Read the model definition and answer for the solid it produces. Units are mm, in the model's axes. A direction names the side the tool comes from. Coordinates: 2 decimals unless noted, no trailing zeros. Order: outer loops, then holes, each group sorted by start corner. A loop starts at its lowest first (then second) coordinate and runs counter-clockwise, first axis right, second up.
```python
from build123d import *

# Parameters (mm, degrees)
F1_DEPTH  = 38.1
F2_DEPTH  = 469.9
F3_DEPTH  = 469.9
F4_DEPTH  = 469.9
F6_DEPTH  = 25.4
F8_DEPTH  = 127
F9_R      = 254
F10_DEPTH = 38.1
F12_DEPTH = 38.1


with BuildPart() as f1:
    # F0 (on Top) → F1 (new body)
    with BuildSketch(Plane.XY):
        Polygon((-164.0508631923, -164.0508649307), (-200.8490917777, -173.9250926458), (-173.9250929642, -200.8490929642), align=None)
        Polygon((-173.9250929642, -200.8490929642), (-200.8490917777, -173.9250926458), (-317.5924246142, -290.6684189572), (-290.6851930936, -317.6091865675), align=None)
        Polygon((-243.6374118769, -14.4661021088), (-200.8490917777, -173.9250926458), (-164.0508631923, -164.0508649307), (-206.8391832914, -4.5918743936), align=None)
        Polygon((-164.0508631923, -164.0508649307), (-173.9250929642, -200.8490929642), (-14.4661048188, -243.6374219761), (-4.5918750468, -206.8391939425), align=None)
        Polygon((-290.6851930936, -317.6091865675), (-317.5924246142, -290.6684189572), (-344.5331937303, -317.6091865675), (-317.6259622097, -344.5499541778), align=None)
        Polygon((-253.5116395921, 22.3321264767), (-243.6374118769, -14.4661021088), (-206.8391832914, -4.5918743936), (-216.7134110066, 32.2063541919), align=None)
        Polygon((-4.5918750468, -206.8391939425), (-14.4661048188, -243.6374219761), (22.3321232148, -253.5116517481), (32.2063529868, -216.7134237145), align=None)
    extrude(amount=-F1_DEPTH)

    # F0 (on Top) → F2 (join)
    with BuildSketch(Plane.XY):
        Polygon((-290.6851930936, -317.6091865675), (-317.5924246142, -290.6684189572), (-344.5331937303, -317.6091865675), (-317.6259622097, -344.5499541778), align=None)
    extrude(amount=F2_DEPTH)

    # F0 (on Top) → F3 (join)
    with BuildSketch(Plane.XY):
        Polygon((-4.5918750468, -206.8391939425), (-14.4661048188, -243.6374219761), (22.3321232148, -253.5116517481), (32.2063529868, -216.7134237145), align=None)
    extrude(amount=F3_DEPTH)

    # F0 (on Top) → F4 (join)
    with BuildSketch(Plane.XY):
        Polygon((-253.5116395921, 22.3321264767), (-243.6374118769, -14.4661021088), (-206.8391832914, -4.5918743936), (-216.7134110066, 32.2063541919), align=None)
    extrude(amount=F4_DEPTH)

    # F5 (on face) → F6 (join)
    with BuildSketch(Plane.XY.offset(469.9)):
        with BuildLine():
            Line((75.3796231443, -162.8212069793), (-156.5023640677, 72.2591707782))
            ThreePointArc((-156.5023640677, 72.2591707782), (-358.8121384382, -359.2018192073), (75.3796231443, -162.8212069793))
        make_face()
    extrude(amount=F6_DEPTH)

    # F7 (on face) → F8 (join)
    with BuildSketch(Plane.XY.offset(495.3)):
        with BuildLine():
            Line((75.3796231443, -162.8212069793), (-199.4597931818, -433.9212904052))
            ThreePointArc((-199.4597931818, -433.9212904052), (0.3896807691, -361.662119627), (75.3796231443, -162.8212069793))
        make_face()
        with BuildLine():
            ThreePointArc((-156.5023640677, 72.2591707782), (-356.3518380185, 0), (-431.3417803937, -198.8409126477))
            Line((-431.3417803937, -198.8409126477), (-156.5023640677, 72.2591707782))
        make_face()
    extrude(amount=F8_DEPTH)

    # F9 (on face) → F10 (join)
    with BuildSketch(Plane.XY.offset(622.3)):
        with Locations((-177.9810786247, -180.8310598135)):
            Circle(F9_R)
    extrude(amount=F10_DEPTH)

    # F11 (on face) → F12 (cut)
    with BuildSketch(Plane.XY.offset(660.4)):
        with BuildLine():
            ThreePointArc((75.3308407052, -162.1476038864), (2.7361824332, -2.3450055803), (-156.1522700542, 72.2292158451))
            Line((-156.1522700542, 72.2292158451), (75.3308407052, -162.1476038864))
        make_face()
    extrude(amount=-F12_DEPTH, mode=Mode.SUBTRACT)


solid = f1.part
```
1) Which of the six approach directions +Z, -Z, +X, -X, +Y, -Y give full straight-line access (tool end or side, diameter ignored) to faces 5 (the flat face through (-244.857, -9.919, 158.27)), 6 (the flat face through (-10.84, -244.61, 158.27)), 7 (the flat face through (-9.46, -224.98, 231.66))?
A:
face 5: -Z, -X
face 6: -Z, -Y
face 7: -X, +Y
2) A cutting plane is placed at A-A, the plane z = 393. Determine the outline of the cut face in (x, y).
A:
outline: (-344.53, -317.61) - (-317.63, -344.55) - (-290.69, -317.61) - (-317.59, -290.67) - close; (-253.51, 22.33) - (-243.64, -14.47) - (-206.84, -4.59) - (-216.71, 32.21) - close; (-14.47, -243.64) - (22.33, -253.51) - (32.21, -216.71) - (-4.59, -206.84) - close
3) Straight lines are drawn through the part: line 1 (Z direction, x = -318.5, y = -339.5); line 2 (Z direction, x = -23, y = -180); line 3 (Z direction, x = 0, y = -273.5). For each, find the intervals that lie inside material, in ascending order.
A:
line 1: z = -38.1 to 495.3, 622.3 to 660.4
line 2: z = 469.9 to 495.3, 622.3 to 660.4
line 3: z = 469.9 to 660.4
4) Determine the mould class of faces 1 (the flat face through (-182, -177, 660.4)), 2 (the flat face through (-295.85, -65.19, 557.91)), 3 (the flat face through (-182, -177, 495.3)), 4 (the flat face through (-38.938, -46.927, 482.422)) for opening direction Z: pulls with the +Z half, pulls with the -Z half, needs draft (parallel to the pull), parting line crosses it, or undercut.
A:
face 1: pulls with the +Z half
face 2: undercut
face 3: undercut
face 4: needs draft
5) A cutting plane is placed at C-C, the plane x = -282.5. Determine the outline of the cut face in (y, z), and give its area (3 significant figures).
A:
outline: (-412.33, 469.9) - (50.67, 469.9) - (50.67, 660.4) - (-412.33, 660.4) - (-412.33, 622.3) - (-52.02, 622.3) - (-52.02, 495.3) - (-412.33, 495.3) - close; (-309.42, -38.1) - (-255.58, -38.1) - (-255.58, 0) - (-309.42, 0) - close
area: 44,500 mm2
6) A cutting plane is placed at D-D, the plane z = 554. Determine the outline of the cut face in (x, y).
A:
outline: (-431.34, -198.84) - (-156.5, 72.26) arc R254 ccw to start; (-199.46, -433.92) arc R254 ccw to (75.38, -162.82) - close
7) Flat-ended cylindrical pins translate along their axes: pin 1 Ø1.5 at (y, z) = (-326.5, 244.5) entering from +X; pin 2 Ø1.5 at (x, z) = (-74.5, 538.5) entering from +Y; pin 3 Ø1.5 at (y, z) = (-324, 405.5) entering from -X. Find the tip coordinate at first contact, or state that the pin passes through.
A:
pin 1: stops at x = -298.83
pin 2: stops at y = -309.92
pin 3: stops at x = -338.9
8) A cutting plane is placed at B-B, the plane y = -226.5. Determine the outline of the cut face in (x, z).
A:
outline: (-427.84, 469.9) - (-9.87, 469.9) - (-9.87, 0) - (-78.33, 0) - (-78.33, -38.1) - (29.58, -38.1) - (29.58, 469.9) - (71.88, 469.9) - (71.88, 660.4) - (-427.84, 660.4) - (-427.84, 622.3) - (10.82, 622.3) - (10.82, 495.3) - (-427.84, 495.3) - close; (-253.42, -38.1) - (-199.58, -38.1) - (-199.58, 0) - (-253.42, 0) - close
